from build123d import *

# Parameters (mm, degrees)
F1_DEPTH  = 15
F3_DEPTH  = 10
F5_DEPTH  = 5
F6_W      = 3.5
F6_H      = 7.5
F7_DEPTH  = 2.5
F8_R      = 2.5
F9_R      = 5
F10_DEPTH = 5


with BuildPart() as f1:
    # F0 (on Front) → F1 (new body)
    with BuildSketch(Plane.XZ):
        Polygon((24.5, 18.5), (-24.5, 18.5), (-28, 18.5), (-28, -18.5), (-24.5, -18.5), (24.5, -18.5), (28, -18.5), (28, 18.5), align=None)
    extrude(amount=F1_DEPTH)

    # F2 (on face) → F3 (cut)
    with BuildSketch(Plane.XZ.offset(15)):
        Polygon((28, 12.5), (24.5, 12.5), (-22, 12.5), (-22, -5.1), (-16, -5.1), (-16, -8.4), (-24.5, -8.4), (-28, -8.4), (-28, -15.9), (-24.5, -15.9), (-1.8, -15.9), (-1.8, -10.7), (-8.1, -10.7), (-8.1, 2.3), (-11, 2.3), (-11, 5.7), (24.5, 5.7), (28, 5.7), align=None)
    extrude(amount=-F3_DEPTH, mode=Mode.SUBTRACT)

    # F4 (on face) → F5 (join)
    with BuildSketch(Plane.XZ.offset(15)):
        Polygon((23, -11.386751), (23, -5.613249), (18, -2.726497), (13, -5.613249), (13, -11.386751), (18, -14.273503), align=None)
    extrude(amount=F5_DEPTH)

    # F6 (on face) → F7 (join)
    with BuildSketch(Plane.XZ.offset(5)):
        with Locations((-26.25, -12.15)):
            Rectangle(F6_W, F6_H)
    extrude(amount=F7_DEPTH)

    # F8
    f8_edges = [f1.edges().sort_by_distance(p)[0] for p in [
        (-28, -7.5, 18.5),
        (28, -7.5, 18.5),
        (28, -7.5, -18.5),
        (-28, -7.5, -18.5),
        (0, 0, -18.5),
        (-28, 0, 0),
        (28, 0, 0),
        (0, 0, 18.5),
    ]]
    fillet(f8_edges, radius=F8_R)

    # F9 (on face) → F10 (join)
    with BuildSketch(Plane.XZ.offset(15)):
        with Locations((5, -5)):
            Circle(F9_R)
    extrude(amount=F10_DEPTH)


solid = f1.part
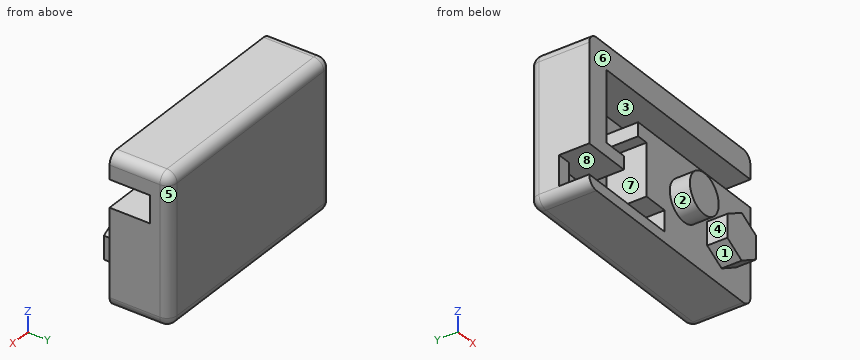
Design review of the part built by this model. Coordinates are the model's own, in mm. Face numbers are marked on the shaded views. A direction names the side the tool comes from. Coordinates: 2 decimals unless noted, no trailing zeros. Loops run counter-clockwise (first coordinate to the right, second up) from the corner with the lowest first, then second, coordinate; pieces in that order, holes last. Notation, with made-up numbers: (60, -16.5) -> (77, -16.5) arc R36 ccw to (77, 22.5) -> close; hole circle Ø5 at (-16.75, 68.25). An arc over 180 degrees is marked (long way). Use a Markdown table: item, result. Add a question column.
Item 1: Wall thickness on L1, parallel to Z at x = -20, y = -6; L2, parallel to Z at x = -6, y = -8.25; L3, parallel to X at y = -8.25, z = -2: over which ranges is each line inside the solid? List them lowest first. Write a range as from..to.
Item 2: We need section D-D, the plane z = 10.5. Write out the cut boundary in (x, y), and give its area (3 significant figures).
Item 3: We need section A-A, the plane y = -11.5. Write out the cut boundary in (x, z).
Item 4: The part is to be moulded in two halves that separate along X. For the marked faces 5, 6, 7 and 8, say which applies: +X half, -X half, draft (parallel to the pull), parting line (faces both ways), or undercut.
Item 5: We need section B-B, the plane z = 4. Write out the cut boundary in (x, y).
Item 6: We need section C-C, the plane x = -19. Write out the cut boundary in (y, z).
Item 7: Machinability: for the marked faces 1, 2, 3 and 4, which of the approach directions +Z, -Z, +X, -X, +Y, -Y give a long, thin tool a straight path to every point of the face, cutting with its end or side? Answer none if there is none.
Item 8: Clearance check with flat-ended pins moving along their axes: P1, Ø10, axis at y = -16.5, z = -6, coming from the +X side; P2, Ø3, axis at x = -5, z = -2.5, coming from the -Y side; P3, Ø2, axis at y = -9, z = 8.5, coming from the +X side; P4, Ø4, axis at x = -27, z = -10.5, coming from the -Y side. State where each tip first meets the part, or that it passes through.
Numbers:
| question | item | result |
|---|---|---|
| 1 | L1 | z = -18.5..-15.9, -8.4..-5.1, 12.5..18.5 |
| 1 | L2 | z = -18.5..-15.9, -10.7..5.7, 12.5..18.5 |
| 1 | L3 | x = -28..-22, -8.1..28 |
| 2 | outline | (-28, -15) -> (-22, -15) -> (-22, -5) -> (28, -5) -> (28, -2.5) arc R2.5 ccw to (25.5, 0) -> (-25.5, 0) arc R2.5 ccw to (-28, -2.5) -> close |
| 2 | area | 337 mm^2 |
| 3 | outline | (-28, -16) arc R2.5 ccw to (-25.5, -18.5) -> (25.5, -18.5) arc R2.5 ccw to (28, -16) -> (28, 5.7) -> (-11, 5.7) -> (-11, 2.3) -> (-8.1, 2.3) -> (-8.1, -10.7) -> (-1.8, -10.7) -> (-1.8, -15.9) -> (-28, -15.9) -> close; (-28, -8.4) -> (-16, -8.4) -> (-16, -5.1) -> (-22, -5.1) -> (-22, 12.5) -> (28, 12.5) -> (28, 16) arc R2.5 ccw to (25.5, 18.5) -> (-25.5, 18.5) arc R2.5 ccw to (-28, 16) -> close |
| 4 | face 5 | +X half |
| 4 | face 6 | draft |
| 4 | face 7 | undercut |
| 4 | face 8 | undercut |
| 5 | outline | (-28, -15) -> (-22, -15) -> (-22, -5) -> (-11, -5) -> (-11, -15) -> (28, -15) -> (28, -2.5) arc R2.5 ccw to (25.5, 0) -> (-25.5, 0) arc R2.5 ccw to (-28, -2.5) -> close |
| 6 | outline | (-15, -18.5) -> (-2.5, -18.5) arc R2.5 ccw to (0, -16) -> (0, 16) arc R2.5 ccw to (-2.5, 18.5) -> (-15, 18.5) -> (-15, 12.5) -> (-5, 12.5) -> (-5, -5.1) -> (-15, -5.1) -> (-15, -8.4) -> (-5, -8.4) -> (-5, -15.9) -> (-15, -15.9) -> close |
| 7 | face 1 | -Z, -X, -Y |
| 7 | face 2 | -Y |
| 7 | face 3 | +X, -Y |
| 7 | face 4 | +Z, -Z, -Y |
| 8 | P1 | stops at x = 28 |
| 8 | P2 | stops at y = -15 |
| 8 | P3 | stops at x = -22 |
| 8 | P4 | stops at y = -7.5 |
